The model under review builds one solid part; all positions refer to its coordinate system, in mm. Face numbers are marked on the shaded views. A direction names the side the tool comes from. Coordinates: 2 decimals unless noted, no trailing zeros. Loops run counter-clockwise (first coordinate to the right, second up) from the corner with the lowest first, then second, coordinate; pieces in that order, holes last. Notation, with made-up numbers: (61.5, 12.25) - (114.5, 12.25) arc R20 ccw to (114.5, 35.25) - close; hole circle Ø8 at (-25, 28). An arc over 180 degrees is marked (long way). Use a Markdown table: item, result. Add a question column.
1) Add section A-A, the plane x = 1.5. Give the boundary of the cut face in (y, z) (3 decimals), and give its area (3 significant figures).
2) The part is to be moulded in two halves that separate along Z. For the marked faces 1, 2 and 3, say which applies: pulls with the +Z half, pulls with the -Z half, needs draft (parallel to the pull), parting line crosses it, or undercut.
3) Add section B-B, the plane y = -7.5. Give the boundary of the cut face in (x, z) (3 decimals), and give its area (3 significant figures).
4) Add section D-D, the plane z = 4.75. Give the boundary of the cut face in (x, y), and give its area (3 significant figures).
5) Add section C-C, the plane x = 4.5. Give the boundary of the cut face in (y, z) (3 decimals), and give its area (3 significant figures).
6) To check wall thickness, follow L1, parallel to Y at x = 1, z = 2.8; L2, parallel to Z at x = 1.75, y = 7.5 (3 decimals); L3, parallel to Y at x = 2.5, z = 2.5 (3 decimals). State the ranges of each line that lie inside material, in increasing order. Write a range as [from, to].
7) For the marked faces 4, 5 and 6, list the 3-axis set-ups (+Z, -Z, +X, -X, +Y, -Y) from which the entire face can be reached by the end or side of a thin tool; tool diameter is ignored.
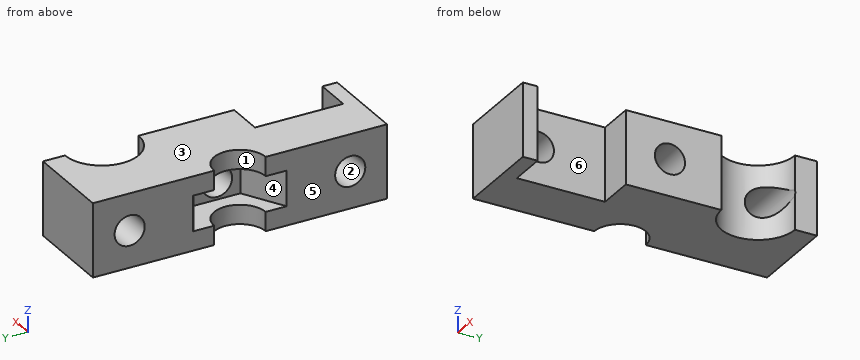
Autodesk Inventor part; units mm, degrees
ref_plane "Work Plane1" through (0, 0, 2.5) normal (0, 0, 1) x (1, 0, 0)
ref_plane "YZ Plane" through (0, 0, 0) normal (1, 0, 0) x (0, 1, 0)
ref_plane "XZ Plane" through (0, 0, 0) normal (0, 1, 0) x (-1, 0, 0)
sketch "Sketch1" plane through (0, 0, 0) normal (0, 0, 1) x (1, 0, 0)
  line L0 (10, -10) -> (-10, -10)
  line L1 (-10, -10) -> (-10, 10)
  line L2 (-10, 10) -> (10, 10)
  line L3 (10, 10) -> (10, -10)
  line L4 (10, -10) -> (-10, 10) construction
  line L5 (-10, -10) -> (10, 10) construction
  line L6 (10, -10) -> (6, -10)
  line L7 (6, -10) -> (6, 10)
  line L8 (6, 10) -> (10, 10)
  line L9 (10, 10) -> (10, -10)
  line L10 (6, 2) -> (4, 2)
  line L11 (4, 2) -> (4, -2)
  line L12 (4, -2) -> (6, -2)
  line L13 (6, -2) -> (6, 2)
  line L14 (0, 10) -> (0, -10)
  point P0 (0, 0)
  dimension "d0" = 20
  dimension "d1" = 20
  dimension "d2" = 4
  dimension "d6" = 2
  dimension "d7" = 2
  dimension "d8" = 4
  dimension "d9" = 2
extrude "Extrusion1" add sketch "Sketch1" along normal blind 5 contours L0 L14 L2 L7 L10 L11 L12
ref_plane "Work Plane1" through (0, 0, 2.5) normal (0, 0, 1) x (1, 0, 0)
sketch "Sketch2" plane through (0, 0, 2.5) normal (0, 0, 1) x (1, 0, 0)
  line L0 (0, 10) -> (0, -10)
  line L1 (0, 3.1754) -> (2.75, 1.5877)
  line L2 (2.75, 1.5877) -> (2.75, -1.5877)
  line L3 (2.75, -1.5877) -> (0, -3.1754)
  line L4 (0, -3.1754) -> (-2.75, -1.5877)
  line L5 (-2.75, -1.5877) -> (-2.75, 1.5877)
  line L6 (-2.75, 1.5877) -> (0, 3.1754)
  point P0 (0, 0)
  point P1 (0, 0)
  dimension "d12" = 5.5
extrude "Extrusion2" cut sketch "Sketch2" along normal mid plane 2.4
sketch "Sketch3" plane through (0, 0, 5) normal (0, 0, 1) x (1, 0, 0)
  circle A0 centre (0, 0) radius 1.75
  dimension "d15" = 3.5
extrude "Extrusion3" cut sketch "Sketch3" against normal blind 8
sketch "Sketch4" plane through (0, 10, 0) normal (-1, 0, 0) x (0, 0, 1)
  circle A0 centre (2.5, -2.5) radius 1.025
  circle A1 centre (2.5, -17.5) radius 1.025
  line L0 (0, 0) -> (5, 0)
  line L1 (0, 0) -> (0, -8.25)
  line L2 (0, -11.75) -> (0, -20)
  line L3 (0, -20) -> (5, -20)
  point P0 (0, -10)
  dimension "d18" = 2.05
  dimension "d19" = 2.05
  dimension "d20" = 2.5
  dimension "d21" = 2.5
  dimension "d22" = 2.5
  dimension "d23" = 2.5
extrude "Extrusion4" cut sketch "Sketch4" against normal blind 25
sketch "Sketch5" plane through (0, 0, 0) normal (0, 0, -1) x (-1, 0, 0)
  line L0 (-6, -2) -> (-4, -2)
  line L1 (-4, -2) -> (-6, -2)
  line L2 (-6, -2) -> (-6, 2)
  line L3 (-6, 2) -> (-4, 2)
  line L4 (-4, 2) -> (-4, -2)
  point P0 (0, 0)
extrude "Extrusion5" add sketch "Sketch5" against normal blind 5
sketch "Sketch6" plane through (0, 0, 0) normal (0, 0, -1) x (-1, 0, 0)
  line L0 (-6, -10) -> (-6, 10)
  circle A0 centre (-6, 6) radius 2.5
  line L1 (-6, -9) -> (-3.5, -9)
  line L2 (-3.5, -9) -> (-3.5, -3)
  line L3 (-3.5, -3) -> (-6, -3)
  line L4 (-6, -3) -> (-6, -9)
  line L5 (0, -10) -> (-6, -10)
  line L6 (-6, 10) -> (0, 10)
  point P0 (0, 0)
  dimension "d32" = 2.5
  dimension "d33" = 1
  dimension "d34" = 6
  dimension "d35" = 5
  dimension "d36" = 4
extrude "Extrusion6" cut sketch "Sketch6" against normal blind 5
sketch "Sketch7" plane through (6, -3, 0) normal (1, 0, 0) x (0, 0, -1)
  circle A0 centre (-2.5, 3) radius 1.025
  line L0 (0, 0) -> (0, 6.5)
  line L1 (0, -7) -> (-5, -7)
  point P0 (0, 3)
  dimension "d39" = 2.5
  dimension "d40" = 10
  dimension "d41" = 2.05
extrude "Extrusion7" cut sketch "Sketch7" against normal blind 20
equation "\"d19\" = d18"
properties part number "POMSliderMotor" material "Acetal Resin, White"
From the geometry:
| question | item | result |
|---|---|---|
| 1 | outline | (-10, 0) - (-0.901, 0) - (-0.901, 1.3) - (-2.309, 1.3) - (-2.309, 3.7) - (-0.901, 3.7) - (-0.901, 5) - (-10, 5) - close; (0.901, 0) - (10, 0) - (10, 5) - (0.901, 5) - (0.901, 3.7) - (2.309, 3.7) - (2.309, 1.3) - (0.901, 1.3) - close; hole circle Ø2.05 at (-7.5, 2.5); hole circle Ø2.05 at (7.5, 2.5) |
| 1 | area | 77.6 mm^2 |
| 2 | face 1 | needs draft |
| 2 | face 2 | undercut |
| 2 | face 3 | pulls with the +Z half |
| 3 | outline | (0, 0) - (3.5, 0) - (3.5, 1.475) - (0, 1.475) - close; (0, 3.525) - (3.5, 3.525) - (3.5, 5) - (0, 5) - close |
| 3 | area | 10.3 mm^2 |
| 4 | outline | (0, -10) - (6, -10) - (6, -9) - (3.5, -9) - (3.5, -3) - (6, -3) - (6, 3.5) arc R2.5 cw to (6, 8.5) - (6, 10) - (0, 10) - (0, 1.75) arc R1.75 cw to (0, -1.75) - close |
| 4 | area | 90.4 mm^2 |
| 5 | outline | (-10, 0) - (-9, 0) - (-9, 5) - (-10, 5) - close; (-3, 0) - (4, 0) - (4, 5) - (-3, 5) - close; (8, 0) - (10, 0) - (10, 5) - (8, 5) - (8, 3.395) arc R1.025 cw to (8, 1.605) - close; hole circle Ø2.05 at (0, 2.5) |
| 5 | area | 46.0 mm^2 |
| 6 | L1 | y = [-10, -8.48], [-6.52, -2.6], [2.6, 6.52], [8.48, 10] |
| 6 | L2 | z = [0, 1.475], [3.525, 5] |
| 6 | L3 | y = [-10, -8.525], [-6.475, -1.732], [1.732, 6.475], [8.525, 10] |
| 7 | face 4 | -X |
| 7 | face 5 | +Z, -Z, -X, +Y, -Y |
| 7 | face 6 | +Z, -Z, +X |
